from build123d import *

# Parameters (mm, degrees)
F1_DEPTH = 10


# Not quite as in the source:
# - ends of sketch curves that miss each other by under 0.0002 mm in the source are joined


with BuildPart() as f1:
    # F0 (on Top) → F1 (new body)
    with BuildSketch(Plane.XY):
        with BuildLine():
            Line((-0.3999973293, 5), (-6.2999973293, 5))
            Line((-6.2999973293, 5), (-6.2999973293, -5))
            Line((-6.2999973293, -5), (6.3, -5))
            Line((6.3, -5), (6.3, 5))
            Line((6.3, 5), (0.4, 5))
            ThreePointArc((0.4, 5), (0.2585786438, 4.9414213562), (0.2, 4.8))
            Line((0.2, 4.8), (0.2, 0))
            ThreePointArc((0.2, 0), (0.1414213562, -0.1414213562), (0, -0.2))
            ThreePointArc((0, -0.2), (-0.1414186856, -0.1414213562), (-0.1999973293, 0))
            Line((-0.1999973293, 0), (-0.1999973293, 4.8))
            ThreePointArc((-0.1999973293, 4.8), (-0.2585759731, 4.9414213562), (-0.3999973293, 5))
        make_face()
    extrude(amount=F1_DEPTH)


solid = f1.part
The listing builds one solid part. Answer for the finished solid, in the listing's coordinates (mm). A direction names the side the tool comes from. Give positions to 0.01 mm unless a question says otherwise; leave off trailing zeros. Write each loop counter-clockwise with the first axis right and the second up, starting at its lowest first coordinate (ties: lowest second). Pieces come first, ordered by that corner, then holes.
Item 1: Section B-B, the plane z = 4.5 is taken. Write down the section's boundary in (x, y).
Item 2: A flat-ended cylindrical pin translates along its axis: P1, Ø3, axis at x = -0.5, y = 1.5, coming from the -Z side. Find the tip coordinate at first contact, or state that the pin passes through.
Item 3: Section A-A, the plane y = 3.75 is taken. Write down the section's boundary in (x, z).
Item 4: Which of the six approach directions +Z, -Z, +X, -X, +Y, -Y give full straight-line access (tool end or side, diameter ignored) to faces 1 (the flat face through (0.2, 2, 5)), 2 (the flat face through (0, -1, 10))?
Item 5: Find the intervals of material crossed by line 1 along X through (y, z) = (0.5, 7.5), in increasing order.
Completed:
1. outline: (-6.3, -5) - (6.3, -5) - (6.3, 5) - (0.4, 5) arc R0.2 ccw to (0.2, 4.8) - (0.2, 0) arc R0.2 cw to (0, -0.2) arc R0.2 cw to (-0.2, 0) - (-0.2, 4.8) arc R0.2 ccw to (-0.4, 5) - (-6.3, 5) - close
2. P1: stops at z = 0
3. outline: (-6.3, 0) - (-0.2, 0) - (-0.2, 10) - (-6.3, 10) - close; (0.2, 0) - (6.3, 0) - (6.3, 10) - (0.2, 10) - close
4. face 1: +Z, -Z, +Y
4. face 2: +Z, +X, -X, +Y, -Y
5. line 1: x = -6.3 to -0.2, 0.2 to 6.3
